```python
from build123d import *

# Parameters (mm, degrees)
F1_DEPTH = 400
F2_R     = 91.560729
F2_R_2   = 60
F3_DEPTH = 400.001
F4_R     = 159.326425
F4_R_2   = 56
F5_DEPTH = 30
F6_R     = 72.9435
F6_R_2   = 56
F7_DEPTH = 30


with BuildPart() as f1:
    # F0 (on Top) → F1 (new body)
    with BuildSketch(Plane.XY):
        Polygon((62.5, -36.084392), (62.5, 36.084392), (0, 72.168784), (-62.5, 36.084392), (-62.5, -36.084392), (0, -72.168784), align=None)
        Polygon((41.136207, 23.75), (41.136207, -23.75), (0, -47.5), (-41.136207, -23.75), (-41.136207, 23.75), (0, 47.5), align=None, mode=Mode.SUBTRACT)
    extrude(amount=F1_DEPTH)

    # F2 (on Top) → F3 (cut, through all)
    with BuildSketch(Plane.XY):
        Circle(F2_R)
        Circle(F2_R_2, mode=Mode.SUBTRACT)
    extrude(amount=F3_DEPTH, mode=Mode.SUBTRACT)

    # F4 (on Top) → F5 (cut)
    with BuildSketch(Plane.XY):
        Circle(F4_R)
        Circle(F4_R_2, mode=Mode.SUBTRACT)
    extrude(amount=F5_DEPTH, mode=Mode.SUBTRACT)

    # F6 (on face) → F7 (cut)
    with BuildSketch(Plane.XY.offset(400)):
        Circle(F6_R)
        Circle(F6_R_2, mode=Mode.SUBTRACT)
    extrude(amount=-F7_DEPTH, mode=Mode.SUBTRACT)


solid = f1.part
```
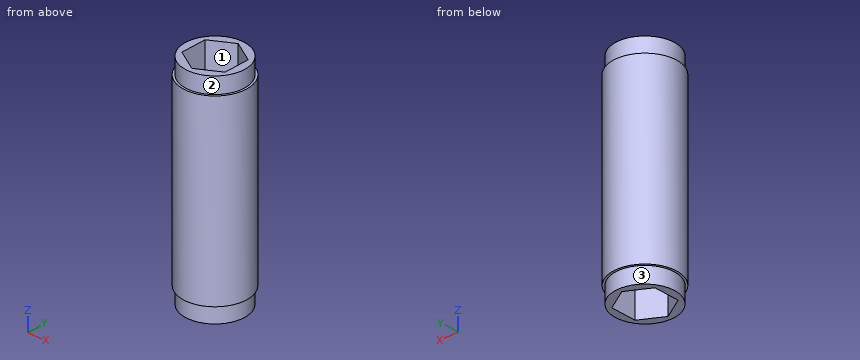
Here's how the part is built. I have some questions about the finished solid (model axes, mm). Face numbers are marked on the shaded views. A direction names the side the tool comes from. Coordinates: 2 decimals unless noted, no trailing zeros. Order: outer loops, then holes, each group sorted by start corner. A loop starts at its lowest first (then second) coordinate and runs counter-clockwise, first axis right, second up. Notation, with made-up numbers: (-19, 5.5) - (29, 5.5) arc R10 ccw to (29, 14.5) - close; hole circle Ø2 at (45.25, 58). An arc over 180 degrees is marked (long way). One line per question, with ' | ' between items. Start each with the question number.
1. Which directions (+Z, -Z, +X, -X, +Y, -Y) give clear straight access to the entire face, cutting with the end or side of a thin tool? Please do the marked faces 1, 2 and 3.
2. If we section it at C-C (x = 20): Write out the boundary of the cut face in (y, z), and give its area (3 significant figures).
3. If we section it at A-A (y = 0): Write out the boundary of the cut face in (x, z), and give its area (3 significant figures).
4. I'm going to push flat-ended pins straight in: pin 1 Ø1.5 at (x, z) = (-10, 251.5) entering from +Y; pin 2 Ø4 at (x, y) = (-44, -21) entering from -Z; pin 3 Ø8 at (y, z) = (25, 146.5) entering from +X (3 decimals); pin 4 Ø1 at (x, z) = (11, 177.5) entering from +Y. Where does each tip first touch, or does it pass through?
5. If we section it at B-B (z = 156.5): Write out the boundary of the cut face in (x, y), and give its area (3 significant figures).
6. If we section it at D-D (x = 47): Write out the boundary of the cut face in (y, z).
7. Please list where these lines run through material, in increasing order: line 1 along X through (y, z) = (-3, 299.5); line 2 along Z through (x, y) = (-47.5, -30); line 3 along Y through (x, z) = (14, 228.5). Write a range as [from, to].
Model answer:
1) face 1: +Z, -Z | face 2: +Z | face 3: -Z
2) outline: (-56.57, 30) - (-52.31, 30) - (-52.31, 0) - (-35.95, 0) - (-35.95, 400) - (-52.31, 400) - (-52.31, 370) - (-56.57, 370) - close; (35.95, 0) - (52.31, 0) - (52.31, 30) - (56.57, 30) - (56.57, 370) - (52.31, 370) - (52.31, 400) - (35.95, 400) - close | area: 16,000 mm²
3) outline: (-60, 30) - (-56, 30) - (-56, 0) - (-41.14, 0) - (-41.14, 400) - (-56, 400) - (-56, 370) - (-60, 370) - close; (41.14, 0) - (56, 0) - (56, 30) - (60, 30) - (60, 370) - (56, 370) - (56, 400) - (41.14, 400) - close | area: 14,600 mm²
4) pin 1: stops at y = 59.28 | pin 2: stops at z = 0 | pin 3: stops at x = 56.205 | pin 4: stops at y = 59.07
5) outline: circle Ø120 at (0, 0); hole (-41.14, -23.75) - (0, -47.5) - (41.14, -23.75) - (41.14, 23.75) - (0, 47.5) - (-41.14, 23.75) - close | area: 5,450 mm²
6) outline: (-37.3, 30) - (-30.45, 30) - (-30.45, 0) - (30.45, 0) - (30.45, 30) - (37.3, 30) - (37.3, 370) - (30.45, 370) - (30.45, 400) - (-30.45, 400) - (-30.45, 370) - (-37.3, 370) - close
7) line 1: x = [-59.92, -41.14], [41.14, 59.92] | line 2: z = [30, 370] | line 3: y = [-58.34, -39.42], [39.42, 58.34]
